The drawing under review shows one solid part. Ordinate dimensions are in mm from its lowest x, y, z. Give positions to 0.01 mm unless a question says otherwise; leave off trailing zeros. Order: outer loops, then holes, each group sorted by start corner. A loop starts at its lowest first (then second) coordinate and runs counter-clockwise, first axis right, second up. Notation, with made-up numbers: (-26.5, -22.75) - (19.5, -22.75) arc R16 ccw to (19.5, -12.75) - close; hole circle Ø1 at (71.5, 70). An arc over 180 degrees is marked (long way). Write item = value, one per line. Start each with the question number.
1. We need section A-A, the plane z = 5.9. Give the boundary of the cut face in (x, y), and give its area (3 significant figures).
2. Mouldability with a two-part tool opening along X and no side actions: class the marked faces 1, 2, 3 and 4 as pulls with the +X half, pulls with the -X half, needs draft (parallel to the pull), parting line crosses it, or undercut.
3. We need section B-B, the plane x = 9.74. Give the boundary of the cut face in (y, z), and give its area (3 significant figures).
4. Wall thickness on probe 1 along X at (y, z) = (3.9, 5.9); probe 2 along Z at (x, y) = (9.25, 1.6); probe 3 along Z at (x, y) = (3.75, 0.7): over which ranges is each line inside the solid? List them lowest first.
5. For P1, Ø3, axis at x = 8.5, z = 12, coming from the +Y side; P2, Ø0.5, axis at y = 2.5, z = 0.5, coming from the -X side; P3, Ø0.5, axis at x = 4.5, z = 0.5, coming from the -Y side (3 decimals), all flat-tipped, find the tip position at first contact; note any pin that passes through.
6. We need section C-C, the plane y = 2.9. Give the boundary of the cut face in (x, z), and give its area (3 significant figures).
7. We need section D-D, the plane z = 14. Give the boundary of the cut face in (x, y) (3 decimals), and give its area (3 significant figures).
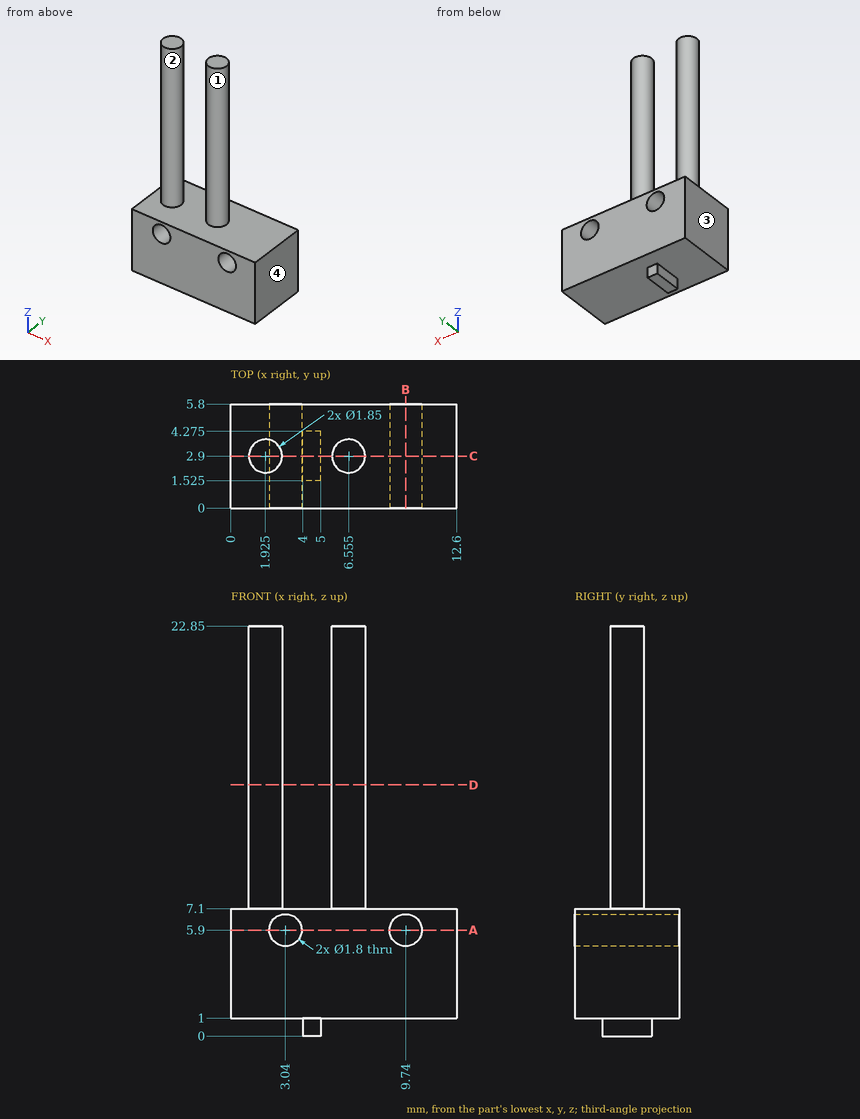
Model answer:
q1.outline = (0, 0) - (2.14, 0) - (2.14, 5.8) - (0, 5.8) - close; (3.94, 0) - (8.84, 0) - (8.84, 5.8) - (3.94, 5.8) - close; (10.64, 0) - (12.6, 0) - (12.6, 5.8) - (10.64, 5.8) - close
q1.area = 52.2 mm2
q2.face_1 = undercut
q2.face_2 = undercut
q2.face_3 = pulls with the -X half
q2.face_4 = pulls with the +X half
q3.outline = (0, 1) - (5.8, 1) - (5.8, 5) - (0, 5) - close; (0, 6.8) - (5.8, 6.8) - (5.8, 7.1) - (0, 7.1) - close
q3.area = 24.9 mm2
q4.probe_1 = 0 to 2.14, 3.94 to 8.84, 10.64 to 12.6
q4.probe_2 = 1 to 5.15, 6.65 to 7.1
q4.probe_3 = 1 to 5.35, 6.45 to 7.1
q5.P1 = 3.71
q5.P2 = 4
q5.P3 = 1.525
q6.outline = (0, 1) - (4, 1) - (4, 0) - (5, 0) - (5, 1) - (12.6, 1) - (12.6, 7.1) - (7.48, 7.1) - (7.48, 22.85) - (5.63, 22.85) - (5.63, 7.1) - (2.85, 7.1) - (2.85, 22.85) - (1, 22.85) - (1, 7.1) - (0, 7.1) - close; hole circle Ø1.8 at (3.04, 5.9); hole circle Ø1.8 at (9.74, 5.9)
q6.area = 131 mm2
q7.outline = circle Ø1.85 at (1.925, 2.9); circle Ø1.85 at (6.555, 2.9)
q7.area = 5.38 mm2
